For this review, use the dimensioned drawing (mm, ordinates from the lowest corner) and the shaded views. A direction names the side the tool comes from. Give positions to 0.01 mm unless a question says otherwise; leave off trailing zeros. Write each loop counter-clockwise with the first axis right and the second up, starting at its lowest first coordinate (ties: lowest second). Pieces come first, ordered by that corner, then holes.
1) We need section A-A on z = 8.5. Give the boundary of the cut face in (x, y), and give its area (4 significant figures).
2) Wall thickness on line 1 along X through (y, z) = (6.25, 6.5); line 2 along Z through (x, y) = (9.5, 2); line 3 along Y through (x, z) = (14.5, 9.5): over which ranges is each line inside the solid? List them lowest first.
3) We need section C-C on x = 3.5. Give the boundary of the cut face in (y, z), and give its area (4 significant figures).
4) For P1, Ø3, axis at x = 12, y = 1.5, coming from the +Z side; P2, Ø1.5, axis at x = 7.5, z = 3, coming from the -Y side, all flat-tipped, find the tip position at first contact; note any pin that passes through.
5) Draft analysis for pull direction X (two halves, no side actions). For the marked faces 1, 2 and 3, state which applies: pulls with the +X half, pulls with the -X half, needs draft (parallel to the pull), parting line crosses it, or undercut.
6) We need section B-B on y = 3.5. Give the boundary of the cut face in (x, z).
7) Machinability: for the marked faces 4 and 5, which of the approach directions +Z, -Z, +X, -X, +Y, -Y give a long, thin tool a straight path to every point of the face, cutting with its end or side? Answer none if there is none.
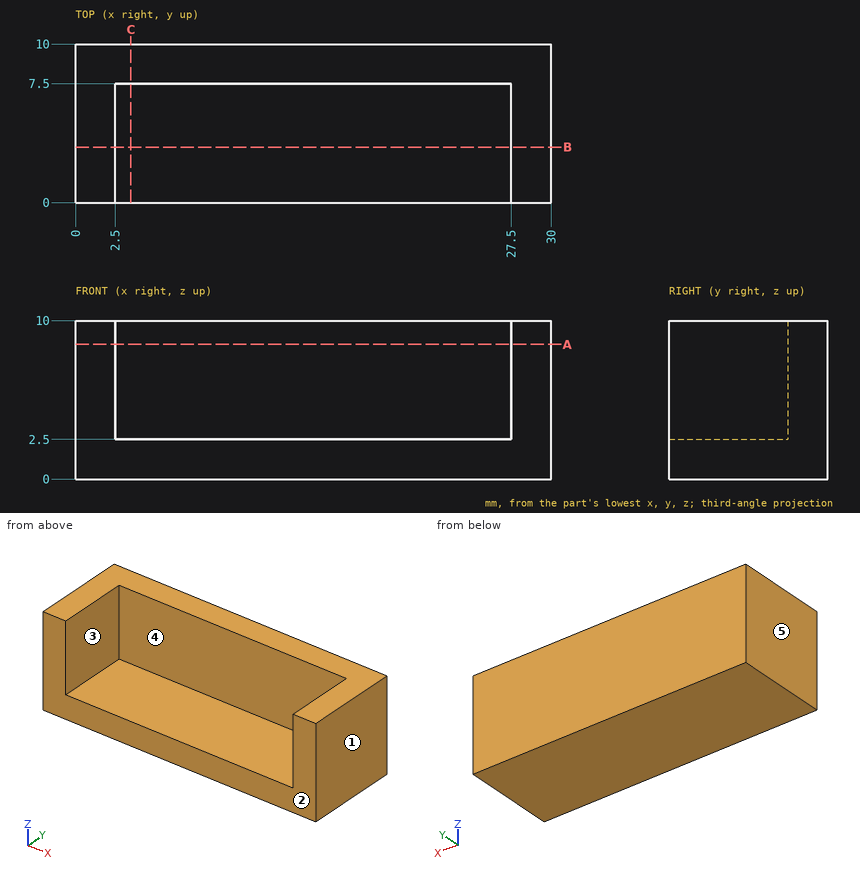
Results list:
1. outline: (0, 0) - (2.5, 0) - (2.5, 7.5) - (27.5, 7.5) - (27.5, 0) - (30, 0) - (30, 10) - (0, 10) - close
1. area: 112.5 mm2
2. line 1: x = 0 to 2.5, 27.5 to 30
2. line 2: z = 0 to 2.5
2. line 3: y = 7.5 to 10
3. outline: (0, 0) - (10, 0) - (10, 10) - (7.5, 10) - (7.5, 2.5) - (0, 2.5) - close
3. area: 43.75 mm2
4. P1: stops at z = 2.5
4. P2: stops at y = 0
5. face 1: pulls with the +X half
5. face 2: needs draft
5. face 3: undercut
6. outline: (0, 0) - (30, 0) - (30, 10) - (27.5, 10) - (27.5, 2.5) - (2.5, 2.5) - (2.5, 10) - (0, 10) - close
7. face 4: +Z, -Y
7. face 5: +Z, -Z, -X, +Y, -Y
